```python
from build123d import *

# Parameters (mm, degrees)
F1_R     = 5.5
F2_DEPTH = 8
F3_R     = 4
F4_DEPTH = 4
F5_R     = 1
F6_DEPTH = 25
F5_R_2   = 2
F7_DEPTH = 5
F8_R     = 5.5
F8_R_2   = 5
F9_DEPTH = 1


with BuildPart() as f2:
    # F1 (on offset) → F2 (new body)
    with BuildSketch(Plane.XY.offset(4)):
        Circle(F1_R)
    extrude(amount=F2_DEPTH)

    # F3 (on face) → F4 (cut)
    with BuildSketch(Plane(origin=(0, 0, 4), x_dir=(1, 0, 0), z_dir=(0, 0, -1))):
        Circle(F3_R)
    extrude(amount=-F4_DEPTH, mode=Mode.SUBTRACT)

    # F5 (on face) → F6 (cut)
    with BuildSketch(Plane.XY.offset(12)):
        Circle(F5_R)
    extrude(amount=-F6_DEPTH, mode=Mode.SUBTRACT)

    # F5 (on face) → F7 (cut)
    with BuildSketch(Plane.XY.offset(12)):
        Circle(F5_R_2)
        Circle(F5_R, mode=Mode.SUBTRACT)
    extrude(amount=-F7_DEPTH, mode=Mode.SUBTRACT)

    # F8 (on face) → F9 (cut)
    with BuildSketch(Plane(origin=(0, 0, 4), x_dir=(1, 0, 0), z_dir=(0, 0, -1))):
        Circle(F8_R)
        Circle(F8_R_2, mode=Mode.SUBTRACT)
    extrude(amount=-F9_DEPTH, mode=Mode.SUBTRACT)


solid = f2.part
```
The listing builds one solid part. Answer for the finished solid, in the listing's coordinates (mm). A direction names the side the tool comes from. Round coordinates to 2 decimals unless told otherwise and drop trailing zeros. Write each loop counter-clockwise with the first axis right and the second up, starting at its lowest first coordinate (ties: lowest second). Pieces come first, ordered by that corner, then holes. Notation, with made-up numbers: (-25.75, 1) -> (-14.75, 1) arc R22 ccw to (-14.75, 36) -> close; hole circle Ø1 at (-12, 54.5). An arc over 180 degrees is marked (long way). Use CSV: the item, a comma, the result in double quotes. Start each with the question number.
(1) Section B-B on x = -1.25 is taken. Give the vertices of the cut face in (y, z), then the cut area to 3 significant figures.
(2) Consider L1, parallel to Y at x = 0, z = 5.15; L2, parallel to Y at x = 0, z = 11.25; L3, parallel to Z at x = 2.5, y = 4.5. Determine where each line is inside the solid, lowest interval first. Write a range as from..to.
(3) Section D-D on x = 4.25 is taken. Give the vertices of the cut face in (y, z).
(4) The mould has two halves that part along Y. Classify faces 1 (the face through (-1.08, 4.88, 4.49)), 2 (the face through (-0.867, 3.905, 5.972)), 3 (the face through (-0.1, -2.4, 12)), 4 (the face through (0, -2, 10)): released by +Y, released by -Y, zero draft, split by the parting line, or undercut.
(5) Which of the six approach directions +Z, -Z, +X, -X, +Y, -Y give full straight-line access (tool end or side, diameter ignored) to faces 5 (the face through (-1.19, -5.37, 8.45)), 6 (the face through (-2, 1, 8))?
(6) Section A-A on y = 0 is taken. Give the vertices of the cut face in (x, z).
(7) Each of these flat-tipped pins is pushed along its axis until it touches: pin 1 (4 mm diameter, centred on x = 4, z = 10, fed in from -Y); pin 2 (4.5 mm diameter, centred on x = 0, y = 0, fed in from -Z); pin 3 (3 mm diameter, centred on y = 3.5, z = 6, fed in from +X). Where does it stop, or does it pass through?
(8) Section C-C on z = 5.5 is taken. Give the vertices of the cut face in (x, y).
A:
1,outline,"(-5.36, 5) -> (-4.84, 5) -> (-4.84, 4) -> (-3.8, 4) -> (-3.8, 8) -> (-1.56, 8) -> (-1.56, 12) -> (-5.36, 12) -> close; (1.56, 8) -> (3.8, 8) -> (3.8, 4) -> (4.84, 4) -> (4.84, 5) -> (5.36, 5) -> (5.36, 12) -> (1.56, 12) -> close"
1,area,"41.8 mm²"
2,L1,"y = -5.5..-4, 4..5.5"
2,L2,"y = -5.5..-2, 2..5.5"
2,L3,"z = 5..12"
3,outline,"(-3.49, 5) -> (-2.63, 5) -> (-2.63, 4) -> (2.63, 4) -> (2.63, 5) -> (3.49, 5) -> (3.49, 12) -> (-3.49, 12) -> close"
4,face 1,"split by the parting line"
4,face 2,"undercut"
4,face 3,"zero draft"
4,face 4,"undercut"
5,face 5,"+Z, -Z"
5,face 6,"-Z"
6,outline,"(-5.5, 5) -> (-5, 5) -> (-5, 4) -> (-4, 4) -> (-4, 8) -> (-2, 8) -> (-2, 12) -> (-5.5, 12) -> close; (2, 8) -> (4, 8) -> (4, 4) -> (5, 4) -> (5, 5) -> (5.5, 5) -> (5.5, 12) -> (2, 12) -> close"
7,pin 1,"stops at y = -5.12"
7,pin 2,"stops at z = 8"
7,pin 3,"stops at x = 5.12"
8,outline,"circle Ø11 at (0, 0); hole circle Ø8 at (0, 0)"
